Could you check a few things on this drawing? It's one solid part, dimensions in mm from its lowest x, y, z. A direction names the side the tool comes from. Round coordinates to 2 decimals unless told otherwise and drop trailing zeros. Write each loop counter-clockwise with the first axis right and the second up, starting at its lowest first coordinate (ties: lowest second). Pieces come first, ordered by that corner, then holes. Notation, with made-up numbers: (15, 84) - (65, 84) arc R27 cw to (65, 102) - close; hole circle Ø8 at (62.5, -1). An arc over 180 degrees is marked (long way). One line per question, with ' | ' between items. Start each with the question number.
(1) If I drill on L1, parallel to X at y = 10, z = 1.4; L2, parallel to Y at x = 10, z = 15.5; L3, parallel to X at y = 6.5, z = 2.5, over which ranges is the centre line in solid material (lowest first)?
(2) Imagine slicing it at B-B (y = 7). Write out the boundary of the cut face in (x, z), plus the area to 3 significant figures.
(3) Will these pins go through, and if not, where does the flat tip stop? pin 1 (4 mm diameter, centred on x = 8.5, z = 2.5, fed in from +Y); pin 2 (4 mm diameter, centred on x = 15.5, z = 15, fed in from +Y); pin 3 (4.5 mm diameter, centred on x = 10, y = 10, fed in from +Z).
(4) Imagine slicing it at D-D (x = 33). Write out the boundary of the cut face in (y, z).
(5) Imagine slicing it at C-C (z = 17.25). Write out the boundary of the cut face in (x, y), plus the area to 3 significant figures.
(6) Imagine slicing it at A-A (x = 10). Write out the boundary of the cut face in (y, z).
(7) Thinking about a two-plate mould opening in X: for the marked faces 1, 2, 3 and 4, which applies, pulls with the +X half, pulls with the -X half, needs draft (parallel to the pull), parting line crosses it, or undercut?
(8) For the marked faces 5, 6 and 7, which set-ups out of +Z, -Z, +X, -X, +Y, -Y let a thin tool reach every point of the face, with its end or its side?
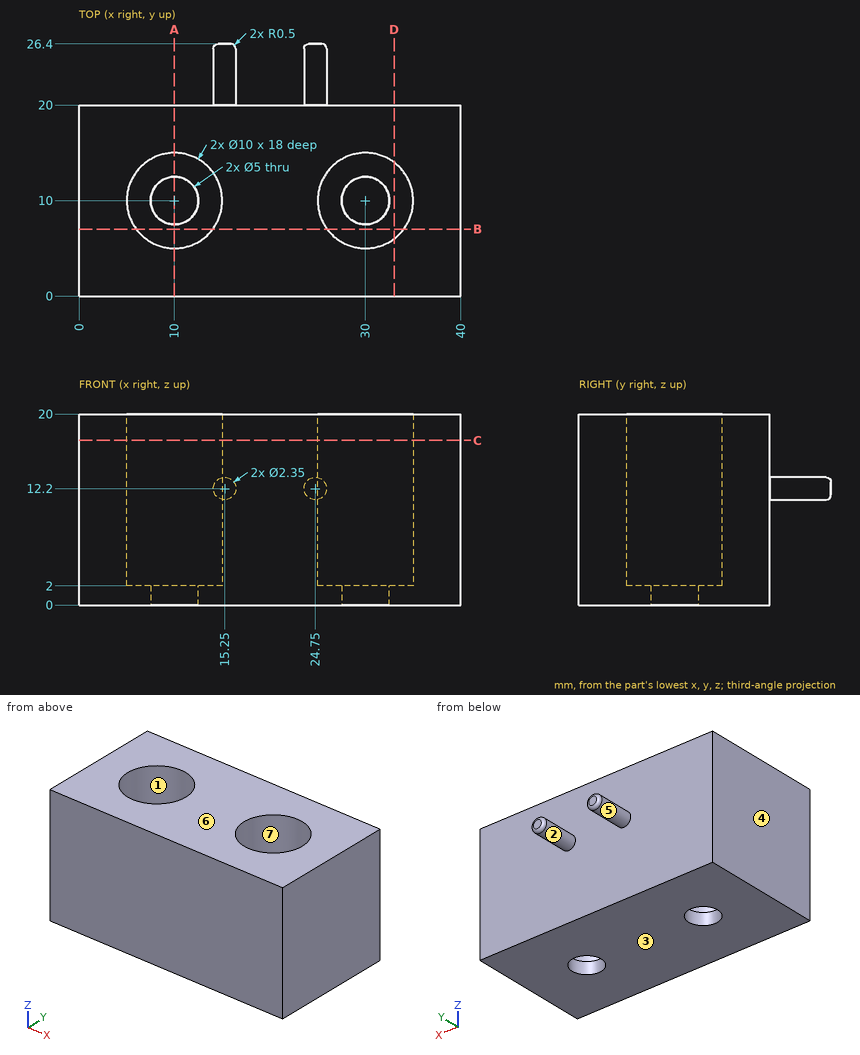
Check sheet entries:
1) L1: 0 to 7.5, 12.5 to 27.5, 32.5 to 40 | L2: 0 to 5, 15 to 20 | L3: 0 to 6.43, 13.57 to 26.43, 33.57 to 40
2) outline: (0, 0) - (40, 0) - (40, 20) - (34, 20) - (34, 2) - (26, 2) - (26, 20) - (14, 20) - (14, 2) - (6, 2) - (6, 20) - (0, 20) - close | area: 512 mm^2
3) pin 1: y = 20 | pin 2: y = 26.38 | pin 3: through
4) outline: (0, 0) - (20, 0) - (20, 20) - (14, 20) - (14, 2) - (6, 2) - (6, 20) - (0, 20) - close
5) outline: (0, 0) - (40, 0) - (40, 20) - (0, 20) - close; hole circle Ø10 at (10, 10); hole circle Ø10 at (30, 10) | area: 643 mm^2
6) outline: (0, 0) - (7.5, 0) - (7.5, 2) - (5, 2) - (5, 20) - (0, 20) - close; (12.5, 0) - (20, 0) - (20, 20) - (15, 20) - (15, 2) - (12.5, 2) - close
7) face 1: undercut | face 2: undercut | face 3: needs draft | face 4: pulls with the -X half
8) face 5: +Y | face 6: +Z, +X, -X, +Y, -Y | face 7: +Z
